```python
from build123d import *

# Parameters (mm, degrees)
F1_DEPTH = 101.6
F3_D     = 4.826
F5_D     = 4.826
F7_D     = 4.826
F9_D     = 4.826


with BuildPart() as f1:
    # F0 (on Right) → F1 (new body)
    with BuildSketch(Plane.YZ):
        with BuildLine():
            Line((-37.30625, 50.8), (-1.5875, 50.8))
            ThreePointArc((-1.5875, 50.8), (-0.464968, 51.264968), (0, 52.3875))
            Line((0, 52.3875), (0, 76.2))
            Line((0, 76.2), (-1.5875, 76.2))
            Line((-1.5875, 76.2), (-1.5875, 53.18125))
            ThreePointArc((-1.5875, 53.18125), (-1.819984, 52.619984), (-2.38125, 52.3875))
            Line((-2.38125, 52.3875), (-38.1, 52.3875))
            ThreePointArc((-38.1, 52.3875), (-39.222532, 51.922532), (-39.6875, 50.8))
            Line((-39.6875, 50.8), (-39.6875, 0))
            Line((-39.6875, 0), (-39.6875, -50.8))
            ThreePointArc((-39.6875, -50.8), (-39.222532, -51.922532), (-38.1, -52.3875))
            Line((-38.1, -52.3875), (-2.38125, -52.3875))
            ThreePointArc((-2.38125, -52.3875), (-1.819984, -52.619984), (-1.5875, -53.18125))
            Line((-1.5875, -53.18125), (-1.5875, -76.2))
            Line((-1.5875, -76.2), (0, -76.2))
            Line((0, -76.2), (0, -52.3875))
            ThreePointArc((0, -52.3875), (-0.464968, -51.264968), (-1.5875, -50.8))
            Line((-1.5875, -50.8), (-37.30625, -50.8))
            ThreePointArc((-37.30625, -50.8), (-37.867516, -50.567516), (-38.1, -50.00625))
            Line((-38.1, -50.00625), (-38.1, 0))
            Line((-38.1, 0), (-38.1, 50.00625))
            ThreePointArc((-38.1, 50.00625), (-37.867516, 50.567516), (-37.30625, 50.8))
        make_face()
    extrude(amount=F1_DEPTH)

    # F3 (through all)
    with Locations(Plane.XZ.offset(1.5875)):
        with Locations((25.4, -64.29375), (76.2, -64.29375)):
            Hole(F3_D / 2)

    # F5 (through all)
    with Locations(Plane.XZ.offset(1.5875)):
        with Locations((25.4, 64.29375), (76.2, 64.29375)):
            Hole(F5_D / 2)

    # F7 (through all)
    with Locations(Plane.XZ.offset(39.6875)):
        with Locations((19.05, 0), (82.55, 0)):
            Hole(F7_D / 2)

    # F9 (through all)
    with Locations(Plane.XZ.offset(39.6875)):
        with Locations((50.8, -31.75), (50.8, 31.75)):
            Hole(F9_D / 2)


solid = f1.part
```
Design review of the part built by this model. Coordinates are the model's own, in mm. A direction names the side the tool comes from. Give positions to 0.01 mm unless a question says otherwise; leave off trailing zeros. Order: outer loops, then holes, each group sorted by start corner. A loop starts at its lowest first (then second) coordinate and runs counter-clockwise, first axis right, second up. Notation, with made-up numbers: (-5, 16.5) -> (49, 16.5) arc R31 cw to (49, 46.5) -> close; hole circle Ø11 at (79, 36). An arc over 180 degrees is marked (long way). Write item = value, one per line. Start each with the question number.
(1) For faces 4 (the face through (50, -1.588, 65)), 5 (the face through (50, -20, -52.388)), 6 (the face through (50, -38.1, -1)), list the 3-axis set-ups (+Z, -Z, +X, -X, +Y, -Y) from which the entire face can be reached by the end or side of a thin tool; tool diameter is ignored.
(2) We need section A-A on z = 0. Write out the cut boundary in (x, y), plus the area to 3 significant figures.
(3) For pin 1 (6.5 mm diameter, centred on x = 76.2, z = -64.29, fed in from -Y); pin 2 (10.5 mm diameter, centred on x = 30.5, y = -27.5, fed in from +Z); pin 3 (8 mm diameter, centred on x = 11.5, z = 8.5, fed in from +Y), all flat-tipped, find the tip position at first contact; note any pin that passes through.
(4) To check wall thickness, follow line 1 along Z through (x, y) = (12, -27); line 2 along Z through (x, y) = (25.4, -0.8); line 3 along Y through (x, z) = (96, 64). State the ranges of each line that lie inside material, in increasing order.
(5) We need section B-B on z = -31.75. Write out the cut boundary in (x, y), plus the area to 3 significant figures.
(6) We need section D-D on y = -8. Write out the cut boundary in (x, z).
(7) We need section C-C on x = 19.05. Write out the cut boundary in (y, z) (1 decimal), plus the area to 3 significant figures.
(8) Mouldability with a two-part tool opening along X and no side actions: class faces 1 (the face through (25.92, -0.78, -66.65)), 2 (the face through (50, -19, -50.8)), 3 (the face through (0, -39, 23)) as +X half, -X half, draft (parallel to the pull), parting line (faces both ways), or undercut.
Numbers:
q1.face_4 = +Z, +X, -X, -Y
q1.face_5 = -Z, +X, -X, -Y
q1.face_6 = +X, -X, +Y
q2.outline = (0, -39.69) -> (16.64, -39.69) -> (16.64, -38.1) -> (0, -38.1) -> close; (21.46, -39.69) -> (80.14, -39.69) -> (80.14, -38.1) -> (21.46, -38.1) -> close; (84.96, -39.69) -> (101.6, -39.69) -> (101.6, -38.1) -> (84.96, -38.1) -> close
q2.area = 146 mm^2
q3.pin_1 = -1.59
q3.pin_2 = 52.39
q3.pin_3 = -38.1
q4.line_1 = -52.39 to -50.8, 50.8 to 52.39
q4.line_2 = -76.2 to -66.71, -61.88 to -51.01, 51.01 to 61.88, 66.71 to 76.2
q4.line_3 = -1.59 to 0
q5.outline = (0, -39.69) -> (48.39, -39.69) -> (48.39, -38.1) -> (0, -38.1) -> close; (53.21, -39.69) -> (101.6, -39.69) -> (101.6, -38.1) -> (53.21, -38.1) -> close
q5.area = 154 mm^2
q6.outline = (0, -52.39) -> (101.6, -52.39) -> (101.6, -50.8) -> (0, -50.8) -> close; (0, 50.8) -> (101.6, 50.8) -> (101.6, 52.39) -> (0, 52.39) -> close
q7.outline = (-39.7, -50.8) arc R1.6 ccw to (-38.1, -52.4) -> (-2.4, -52.4) arc R0.8 cw to (-1.6, -53.2) -> (-1.6, -76.2) -> (0, -76.2) -> (0, -52.4) arc R1.6 ccw to (-1.6, -50.8) -> (-37.3, -50.8) arc R0.8 cw to (-38.1, -50) -> (-38.1, -2.4) -> (-39.7, -2.4) -> close; (-39.7, 2.4) -> (-38.1, 2.4) -> (-38.1, 50) arc R0.8 cw to (-37.3, 50.8) -> (-1.6, 50.8) arc R1.6 ccw to (0, 52.4) -> (0, 76.2) -> (-1.6, 76.2) -> (-1.6, 53.2) arc R0.8 cw to (-2.4, 52.4) -> (-38.1, 52.4) arc R1.6 ccw to (-39.7, 50.8) -> close
q7.area = 354 mm^2
q8.face_1 = undercut
q8.face_2 = draft
q8.face_3 = -X half
